Geometry: final body of the model. Coordinates: model frame, mm. Face numbers are marked on the shaded views. A direction names the side the tool comes from. Coordinates: 2 decimals unless noted, no trailing zeros. Write item = value, one per line. Start each with the question number.
Item 1: Reachability of the marked faces 1 and 2 from +Z, -Z, +X, -X, +Y, -Y: full face, straight path, thin tool, end or side. Return the list, or none.
Item 2: Ray query, L1, parallel to Y at x = 0, z = 20; L2, parallel to Y at x = -18.5, z = 26; L3, parallel to X at y = 82.5, z = 22. Return the intervals inside material, ascending. Write a range as [from, to].
Item 3: Section A-A on y = 0. Give the number of separate pieces and of enclosed holes in the cut face, plus the area to 3 significant figures.
Item 4: First-contact query: pin 1 Ø2 at (x, y) = (17, 90) entering from +Z; pin 2 Ø5 at (y, z) = (-92.5, 6.5) entering from +X; pin 3 Ø8 at (y, z) = (-15, -1.5) entering from +X. Flat tips, straight axial feed; report the tip coordinate or a pass-through.
Item 5: Pull-direction query (X, two-part tool) for the marked faces 3 and 4; classes: +X half, -X half, draft (parallel to the pull), parting line (faces both ways), or undercut.
Autodesk Inventor part; units mm, degrees
ref_plane "YZ Plane" through (0, 0, 0) normal (1, 0, 0) x (0, 1, 0)
ref_plane "XZ Plane" through (0, 0, 0) normal (0, 1, 0) x (-1, 0, 0)
ref_plane "XY Plane" through (0, 0, 0) normal (0, 0, 1) x (1, 0, 0)
sketch "Sketch1" plane through (0, 0, 0) normal (0, 0, 1) x (1, 0, 0)
  line L0 (70.3905, -134.62) -> (-70.3905, -134.62)
  line L1 (-81.3891, -128.27) -> (-151.7796, -6.35)
  line L2 (-151.7796, 6.35) -> (-81.3891, 128.27)
  line L3 (-70.3905, 134.62) -> (70.3905, 134.62)
  line L4 (81.3891, 128.27) -> (151.7796, 6.35)
  line L5 (151.7796, -6.35) -> (81.3891, -128.27)
  arc A0 (-70.3905, 134.62) -> (-81.3891, 128.27) centre (-70.3905, 121.92) ccw
  arc A1 (-151.7796, 6.35) -> (-151.7796, -6.35) centre (-140.7811, 0) ccw
  arc A2 (-81.3891, -128.27) -> (-70.3905, -134.62) centre (-70.3905, -121.92) ccw
  arc A3 (70.3905, -134.62) -> (81.3891, -128.27) centre (70.3905, -121.92) ccw
  arc A4 (151.7796, -6.35) -> (151.7796, 6.35) centre (140.7811, 0) ccw
  arc A5 (81.3891, 128.27) -> (70.3905, 134.62) centre (70.3905, 121.92) ccw
  point P0 (0, 0)
  point P1 (0, 0)
  point P2 (77.7229, -134.62)
  point P3 (-77.7229, -134.62)
  point P4 (-155.4458, 0)
  point P5 (-77.7229, 134.62)
  point P6 (77.7229, 134.62)
  point P7 (155.4458, 0)
  dimension "d0" = 269.24
  dimension "d1" = 12.7
extrude "Extrusion1" add sketch "Sketch1" along normal blind 15.24
sketch "Sketch2" plane through (0, 0, 15.24) normal (0, 0, 1) x (1, 0, 0)
  circle A0 centre (0, 0) radius 17.78
  circle A1 centre (0, 0) radius 58.42
  dimension "d5" = 35.56
  dimension "d8" = 116.84
extrude "Extrusion2" cut sketch "Sketch2" against normal through all contours A0
sketch "Sketch3" plane through (0, 0, 0) normal (0, 0, -1) x (-1, 0, 0)
  circle A0 centre (0, 0) radius 17.78
  circle A1 centre (0, 0) radius 58.42
  dimension "d9" = 116.84
extrude "Extrusion3" add sketch "Sketch3" along normal blind 10.16
fillet "Fillet1" radius 10.16 1 edges at (58.42, 0, 0)
fillet "Fillet2" radius 5.08 12 edges at (-76.7405, 132.9185, 0) (-116.5843, 67.31, 0) (-153.4811, 0, 0) (-116.5843, -67.31, 0) (-76.7405, -132.9185, 0) (0, -134.62, 0) (76.7405, -132.9185, 0) (116.5843, -67.31, 0) (153.4811, 0, 0) (116.5843, 67.31, 0) (76.7405, 132.9185, 0) (0, 134.62, 0)
sketch "Sketch4" plane through (0, 0, 15.24) normal (0, 0, 1) x (1, 0, 0)
  circle A0 centre (0, 0) radius 129.54 construction
  circle A1 centre (0, 0) radius 35.56
  circle A2 centre (0, 0) radius 48.26
  circle A3 centre (0, 0) radius 17.78
  circle A4 centre (0, 0) radius 101.6
  circle A5 centre (0, 0) radius 114.3
  circle A6 centre (-129.54, 0) radius 8.89
  circle A7 centre (-64.77, -112.1849) radius 8.89
  circle A8 centre (64.77, -112.1849) radius 8.89
  circle A9 centre (129.54, 0) radius 8.89
  circle A10 centre (64.77, 112.1849) radius 8.89
  circle A11 centre (-64.77, 112.1849) radius 8.89
  dimension "d14" = 259.08
  dimension "d15" = 71.12
  dimension "d16" = 96.52
  dimension "d17" = 203.2
  dimension "d18" = 228.6
  dimension "d19" = 17.78
  dimension "d22" = 360
extrude "Extrusion4" add sketch "Sketch4" along normal blind 15.24 contours A2 | A5
extrude "Extrusion5" cut sketch "Sketch4" against normal through all contours A6 | A7 | A8 | A9 | A10 | A11
fillet "Fillet3" radius 5.08 2 edges at (-101.6, 0, 15.24) (-48.26, 0, 15.24)
chamfer "Chamfer1" distance 2.54 angle 45 1 edges at (-114.3, 0, 30.48)
equation "\"BendRadius\" = Thickness"
equation "\"BendReliefWidth\" = Thickness"
equation "\"BendReliefDepth\" = 0.5 * Thickness"
equation "\"CornerReliefSize\" = 4 * Thickness"
equation "\"MinimumRemnant\" = 2 * Thickness"
equation "\"TransitionRadius\" = BendRadius"
equation "\"JacobiRadiusSize\" = BendRadius"
equation "\"GapSize\" = Thickness"
properties part number "crank case cover" material "Aluminum 6061"
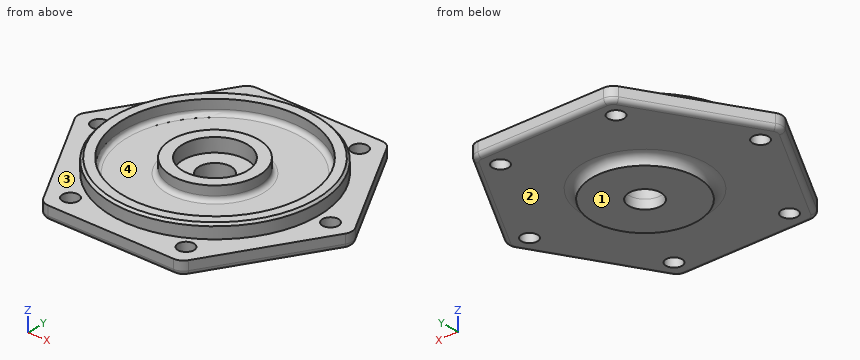
Responses:
q1.face_1 = -Z, +X, -X, +Y, -Y
q1.face_2 = -Z
q2.L1 = [-114.3, -101.59], [-48.27, -35.56], [35.56, 48.27], [101.59, 114.3]
q2.L2 = [-112.79, -99.9], [-44.57, -30.37], [30.37, 44.57], [99.9, 112.79]
q2.L3 = [-79.11, -59.3], [59.3, 79.11]
q3.separate_pieces = 4
q3.enclosed_holes = 0
q3.area = 5,240 mm²
q4.pin_1 = 15.24
q4.pin_2 = 103.48
q4.pin_3 = 146.71
q5.face_3 = draft
q5.face_4 = undercut
